```python
from build123d import *

# Parameters (mm, degrees)
F0_W     = 69.5
F0_H     = 23
F1_DEPTH = 1.5
F0_W_2   = 1
F0_H_2   = 4
F2_DEPTH = 10
F4_DEPTH = 69.501


with BuildPart() as f1:
    # F0 (on Top) → F1 (new body)
    with BuildSketch(Plane.XY):
        with Locations((3.447164, -3.000336)):
            Rectangle(F0_W, F0_H)
        Polygon((-29.802836, -13.000336), (-29.802836, 6.999664), (-15.802836, 6.999664), (-14.802836, 6.999664), (-13.302836, 6.999664), (-12.302836, 6.999664), (1.697164, 6.999664), (2.697164, 6.999664), (4.197164, 6.999664), (5.197164, 6.999664), (19.197164, 6.999664), (20.197164, 6.999664), (21.697164, 6.999664), (22.697164, 6.999664), (36.697164, 6.999664), (36.697164, -13.000336), (22.697164, -13.000336), (21.697164, -13.000336), (20.197164, -13.000336), (19.197164, -13.000336), (5.197164, -13.000336), (4.197164, -13.000336), (2.697164, -13.000336), (1.697164, -13.000336), (-12.302836, -13.000336), (-13.302836, -13.000336), (-14.802836, -13.000336), (-15.802836, -13.000336), align=None, mode=Mode.SUBTRACT)
    extrude(amount=F1_DEPTH)

    # F0 (on Top) → F2 (join)
    with BuildSketch(Plane.XY):
        with Locations((3.447164, -3.000336)):
            Rectangle(F0_W, F0_H)
        Polygon((-29.802836, -13.000336), (-29.802836, 6.999664), (-15.802836, 6.999664), (-14.802836, 6.999664), (-13.302836, 6.999664), (-12.302836, 6.999664), (1.697164, 6.999664), (2.697164, 6.999664), (4.197164, 6.999664), (5.197164, 6.999664), (19.197164, 6.999664), (20.197164, 6.999664), (21.697164, 6.999664), (22.697164, 6.999664), (36.697164, 6.999664), (36.697164, -13.000336), (22.697164, -13.000336), (21.697164, -13.000336), (20.197164, -13.000336), (19.197164, -13.000336), (5.197164, -13.000336), (4.197164, -13.000336), (2.697164, -13.000336), (1.697164, -13.000336), (-12.302836, -13.000336), (-13.302836, -13.000336), (-14.802836, -13.000336), (-15.802836, -13.000336), align=None, mode=Mode.SUBTRACT)
        with Locations((-15.302836, -11.000336)):
            Rectangle(F0_W_2, F0_H_2)
        with Locations((-12.802836, -11.000336)):
            Rectangle(F0_W_2, F0_H_2)
        with Locations((2.197164, -11.000336)):
            Rectangle(F0_W_2, F0_H_2)
        with Locations((4.697164, -11.000336)):
            Rectangle(F0_W_2, F0_H_2)
        with Locations((19.697164, -11.000336)):
            Rectangle(F0_W_2, F0_H_2)
        with Locations((22.197164, -11.000336)):
            Rectangle(F0_W_2, F0_H_2)
        with Locations((22.197164, 4.999664)):
            Rectangle(F0_W_2, F0_H_2)
        with Locations((19.697164, 4.999664)):
            Rectangle(F0_W_2, F0_H_2)
        with Locations((4.697164, 4.999664)):
            Rectangle(F0_W_2, F0_H_2)
        with Locations((2.197164, 4.999664)):
            Rectangle(F0_W_2, F0_H_2)
        with Locations((-12.802836, 4.999664)):
            Rectangle(F0_W_2, F0_H_2)
        with Locations((-15.302836, 4.999664)):
            Rectangle(F0_W_2, F0_H_2)
    extrude(amount=-F2_DEPTH)

    # F3 (on face) → F4 (cut, through all)
    with BuildSketch(Plane(origin=(-31.302836, 0, 0), x_dir=(0, -1, 0), z_dir=(-1, 0, 0))):
        with BuildLine():
            Line((0.500336, -5), (0.500336, -10))
            Line((0.500336, -10), (5.500336, -10))
            Line((5.500336, -10), (5.500336, -5))
            ThreePointArc((5.500336, -5), (3.000336, -2.5), (0.500336, -5))
        make_face()
    extrude(amount=-F4_DEPTH, mode=Mode.SUBTRACT)


solid = f1.part
```
Here's how the part is built. I have some questions about the finished solid (model axes, mm). A direction names the side the tool comes from. Coordinates: 2 decimals unless noted, no trailing zeros. Order: outer loops, then holes, each group sorted by start corner. A loop starts at its lowest first (then second) coordinate and runs counter-clockwise, first axis right, second up.
1) Imagine slicing it at C-C on y = 4.25. State how many separate pieces and enclosed holes the cut face has, and give its area (3 significant figures).
2) Which directions (+Z, -Z, +X, -X, +Y, -Y) give clear straight access to the entire face, cutting with the end or side of a thin tool? Please do faces 1 (the face through (-31, -5.5, -8)), 2 (the face through (38.197, -3, -2)), 3 (the face through (22.697, -11, -5)).
3) Will these pins go through, and if not, where does the flat tip stop? pin 1 (0.5 mm diameter, centred on x = 2.5, y = 5, fed in from +Z); pin 2 (5 mm diameter, centred on x = 16, y = 1.5, fed in from +Z).
4) Imagine slicing it at B-B on y = -8. List the corners of the cut face in (x, z) for me.
5) Imagine slicing it at A-A on x = -9.5. List the corners of the cut face in (y, z) for me, and give its area (3 significant figures).
6) We'd pull the mould along Y, two halves only. Please class faces 4 (the face through (3, -14, -10)), 5 (the face through (-15.803, 5, -5)): +Y half, -Y half, draft (parallel to the pull), parting line (faces both ways), or undercut.
7) I need wall thicknesses on line 1 (Y direction, x = 33, z = -6); line 2 (X direction, y = -1, z = 1); line 3 (Y direction, x = 20, z = -5.25). Which ranges of each line are inside material? Lowest first, please.
Response values:
1. separate pieces: 8
1. enclosed holes: 0
1. area: 94.5 mm2
2. face 1: -Z, +X, -X
2. face 2: +Z, -Z, +X, +Y, -Y
2. face 3: +Z, -Z
3. pin 1: stops at z = 0
3. pin 2: passes through
4. outline: (-31.3, -10) - (-29.8, -10) - (-29.8, 1.5) - (-31.3, 1.5) - close; (36.7, -10) - (38.2, -10) - (38.2, 1.5) - (36.7, 1.5) - close
5. outline: (-14.5, -10) - (-13, -10) - (-13, 1.5) - (-14.5, 1.5) - close; (7, -10) - (8.5, -10) - (8.5, 1.5) - (7, 1.5) - close
5. area: 34.5 mm2
6. face 4: draft
6. face 5: undercut
7. line 1: y = -14.5 to -13, 7 to 8.5
7. line 2: x = -31.3 to -29.8, 36.7 to 38.2
7. line 3: y = -14.5 to -9, 3 to 8.5
